```python
from build123d import *

# Parameters (mm, degrees)
SCHIZZO1_R                                           = 4.2
SCHIZZO1_R_2                                         = 2.61831532
ESTRUSIONE_ESTRUSIONE1_DEPTH                         = 10
TAGLIO_ESTRUSIONE1_DEPTH                             = 6.5
SCHIZZO3_R                                           = 3.5
SCHIZZO3_R_2                                         = 3
TAGLIO_ESTRUSIONE2_DEPTH                             = 6.5
FORO_LAMATO_PER_VITE_M8_A_TESTA_CILINDRI_D           = 9
FORO_LAMATO_PER_VITE_M8_A_TESTA_CILINDRI_CBORE_D     = 15
FORO_LAMATO_PER_VITE_M8_A_TESTA_CILINDRI_CBORE_DEPTH = 5


with BuildPart() as part:
    # Schizzo1 → Estrusione-Estrusione1 (new body)
    with BuildSketch(Plane.XY):
        Polygon((0, 0), (95, 0), (95, 246), (81, 260), (14, 260), (0, 246), align=None)
        with Locations((22.770722004, 10)):
            Circle(SCHIZZO1_R, mode=Mode.SUBTRACT)
        with Locations((47.5, 10)):
            Circle(SCHIZZO1_R, mode=Mode.SUBTRACT)
        with Locations(Location((72.229277996, 10, 0), (0, 0, 180))):
            Circle(SCHIZZO1_R, mode=Mode.SUBTRACT)
        with Locations((4, 163.3)):
            Circle(SCHIZZO1_R_2, mode=Mode.SUBTRACT)
        with Locations((30, 163.3)):
            Circle(SCHIZZO1_R_2, mode=Mode.SUBTRACT)
        with Locations(Location((65, 163.3, 0), (0, 0, 180))):
            Circle(SCHIZZO1_R_2, mode=Mode.SUBTRACT)
        with Locations(Location((91, 163.3, 0), (0, 0, 180))):
            Circle(SCHIZZO1_R_2, mode=Mode.SUBTRACT)
        with Locations((91, 197.3)):
            Circle(SCHIZZO1_R_2, mode=Mode.SUBTRACT)
        with Locations((65, 197.3)):
            Circle(SCHIZZO1_R_2, mode=Mode.SUBTRACT)
        with Locations(Location((30, 197.3, 0), (0, 0, 180))):
            Circle(SCHIZZO1_R_2, mode=Mode.SUBTRACT)
        with Locations(Location((4, 197.3, 0), (0, 0, 180))):
            Circle(SCHIZZO1_R_2, mode=Mode.SUBTRACT)
    extrude(amount=-ESTRUSIONE_ESTRUSIONE1_DEPTH)

    # Schizzo2 → Taglio-Estrusione1 (cut)
    with BuildSketch(Plane.XY):
        with BuildLine():
            Line((25.504353305, 260), (25.504353305, 219))
            ThreePointArc((25.504353305, 219), (26.383032962, 216.878679656), (28.504353305, 216))
            Line((28.504353305, 216), (66.495646695, 216))
            ThreePointArc((66.495646695, 216), (68.616967038, 216.878679656), (69.495646695, 219))
            Line((69.495646695, 219), (69.495646695, 260))
            Line((69.495646695, 260), (25.504353305, 260))
        make_face()
    extrude(amount=-TAGLIO_ESTRUSIONE1_DEPTH, mode=Mode.SUBTRACT)

    # Schizzo3 → Taglio-Estrusione2 (cut)
    with BuildSketch(Plane.XY.offset(-6.5)):
        with Locations((33.5, 253)):
            Circle(SCHIZZO3_R)
        with Locations((33.5, 240)):
            Circle(SCHIZZO3_R_2)
        with Locations((61.5, 240)):
            Circle(SCHIZZO3_R_2)
        with Locations((61.5, 227)):
            Circle(SCHIZZO3_R)
    extrude(amount=-TAGLIO_ESTRUSIONE2_DEPTH, mode=Mode.SUBTRACT)

    # Foro lamato per Vite M8 a testa cilindrica piana-1 (through all)
    with Locations(Plane(origin=(47.5, 10, 0), x_dir=(1, 0, 0), z_dir=(0, 0, 1))):
        with Locations((0, 0), (-24.729277996, 0), (24.729277996, 0)):
            CounterBoreHole(FORO_LAMATO_PER_VITE_M8_A_TESTA_CILINDRI_D / 2, FORO_LAMATO_PER_VITE_M8_A_TESTA_CILINDRI_CBORE_D / 2, FORO_LAMATO_PER_VITE_M8_A_TESTA_CILINDRI_CBORE_DEPTH)


solid = part.part
```
CAD build for the part. Positions are in the model's coordinates, mm. A direction names the side the tool comes from. Coordinates: 2 decimals unless noted, no trailing zeros. Loops run counter-clockwise (first coordinate to the right, second up) from the corner with the lowest first, then second, coordinate; pieces in that order, holes last. Notation, with made-up numbers: (78, -34.5) - (126, -34.5) arc R31 ccw to (126, -7.5) - close; hole circle Ø8 at (-28.5, 42). An arc over 180 degrees is marked (long way). Use CSV: the item, a comma, the result in double quotes. Start each with the question number.
Q1. Cut at D-D, the plane z = -2. State how many separate pieces and enclosed holes the cut face has, then the cut area to 3 significant figures.
Q2. Probe probe 1 along X at (y, z) = (163.3, -5.75); probe 2 along Y at (x, z) = (30, -6.25); probe 3 along Y at (x, z) = (61.5, -8.3). List the from-to ranges inside material, lowest first. Write a range as from..to.
Q3. Cut at B-B, the plane y = 10. List the corners of the cut face in (x, z), then the cut area to 3 significant figures.
Q4. 3-axis set-ups, long thin cutter, end or side, ignore diameter. For faces 1 (the flat face through (0, 125, -5)), 2 (the flat face through (47, 5, -5)), 3 (the flat face through (47, 216, -3)): which of +Z, -Z, +X, -X, +Y, -Y reach the whole face in a straight line?
Q5. Two-plate mould, pull along Y, no slides. Class faces 4 (the cylindrical face through (61.04, 230.47, -8.23)), 5 (the flat face through (47, 132, -10)), 6 (the flat face through (48, 260, -7)): +Y half, -Y half, draft (parallel to the pull), parting line (faces both ways), or undercut.
Q6. Drop flat-ended pins along their axis: P1, Ø3, axis at x = 85, z = -7.5, coming from the +Y side; P2, Ø4, axis at x = 61.5, z = -2, coming from the +Y side; P3, Ø8, axis at x = 33.5, y = 253, coming from the +Z side. Give the stop position or say it passes through.
Q7. Cut at A-A, the plane y = 240. List the corners of the cut face in (x, z).
Q8. Cut at C-C, the plane x = 91. List the corners of the cut face in (y, z).
Here are the results:
1,separate pieces,"1"
1,enclosed holes,"11"
1,area,"21,900 mm2"
2,probe 1,"0..1.38, 6.62..27.38, 32.62..62.38, 67.62..88.38, 93.62..95"
2,probe 2,"0..160.68, 165.92..194.68, 199.92..216"
2,probe 3,"0..223.5, 230.5..237, 243..260"
3,outline,"(0, -10) - (18.27, -10) - (18.27, -5) - (15.27, -5) - (15.27, 0) - (0, 0) - close; (27.27, -10) - (43, -10) - (43, -5) - (40, -5) - (40, 0) - (30.27, 0) - (30.27, -5) - (27.27, -5) - close; (52, -10) - (67.73, -10) - (67.73, -5) - (64.73, -5) - (64.73, 0) - (55, 0) - (55, -5) - (52, -5) - close; (76.73, -10) - (95, -10) - (95, 0) - (79.73, 0) - (79.73, -5) - (76.73, -5) - close"
3,area,"590 mm2"
4,face 1,"+Z, -Z, -X, +Y, -Y"
4,face 2,"+Z"
4,face 3,"+Z, +Y"
5,face 4,"undercut"
5,face 5,"draft"
5,face 6,"+Y half"
6,P1,"y = 257.5"
6,P2,"y = 216"
6,P3,"z = -6.5"
7,outline,"(0, -10) - (30.5, -10) - (30.5, -6.5) - (25.5, -6.5) - (25.5, 0) - (0, 0) - close; (36.5, -10) - (58.5, -10) - (58.5, -6.5) - (36.5, -6.5) - close; (64.5, -10) - (95, -10) - (95, 0) - (69.5, 0) - (69.5, -6.5) - (64.5, -6.5) - close"
8,outline,"(0, -10) - (160.68, -10) - (160.68, 0) - (0, 0) - close; (165.92, -10) - (194.68, -10) - (194.68, 0) - (165.92, 0) - close; (199.92, -10) - (250, -10) - (250, 0) - (199.92, 0) - close"
